Geometry: final body of the model. Coordinates: model frame, mm. Give positions to 0.01 mm unless a question says otherwise; leave off trailing zeros. Write each loop counter-clockwise with the first axis right and the second up, starting at its lowest first coordinate (ties: lowest second). Pieces come first, ordered by that corner, then holes. Notation, with made-up numbers: (-19, 68) -> (33, 68) arc R27 cw to (33, 84) -> close; hole circle Ø3 at (-16.5, 31.25). An arc over 180 degrees is marked (long way). Answer as a JSON object with one key per item and string values.
from build123d import *

# Parameters (mm, degrees)
SKETCH_1_R      = 1.5
EXTRUDE_1_DEPTH = 3


with BuildPart() as part:
    # 草图1 → 凸台-拉伸1 (new body)
    with BuildSketch(Plane.XY):
        with BuildLine():
            Line((116, -441), (116, -336.18))
            ThreePointArc((116, -336.18), (118, -332.18), (116, -328.18))
            Line((116, -328.18), (116, -4))
            ThreePointArc((116, -4), (116.535533906, 3.535533906), (109, 3))
            Line((109, 3), (106, 3))
            Line((106, 3), (106, -21.645755349))
            Line((106, -21.645755349), (7, -21.645755349))
            Line((7, -21.645755349), (7, 3))
            Line((7, 3), (4, 3))
            ThreePointArc((4, 3), (-3.535533906, 3.535533906), (-3, -4))
            Line((-3, -4), (-3, -328.18))
            ThreePointArc((-3, -328.18), (-5, -332.18), (-3, -336.18))
            Line((-3, -336.18), (-3, -441))
            ThreePointArc((-3, -441), (-3.535533906, -448.535533906), (4, -448))
            Line((4, -448), (109, -448))
            ThreePointArc((109, -448), (116.535533906, -448.535533906), (116, -441))
        make_face()
        Circle(SKETCH_1_R, mode=Mode.SUBTRACT)
        with Locations((113, 0)):
            Circle(SKETCH_1_R, mode=Mode.SUBTRACT)
        with Locations((113, -445)):
            Circle(SKETCH_1_R, mode=Mode.SUBTRACT)
        with Locations((0, -445)):
            Circle(SKETCH_1_R, mode=Mode.SUBTRACT)
        with Locations((0, -332.18)):
            Circle(SKETCH_1_R, mode=Mode.SUBTRACT)
        with Locations((113, -332.18)):
            Circle(SKETCH_1_R, mode=Mode.SUBTRACT)
        with BuildLine():
            Line((101, -37), (101, -353.3033361))
            ThreePointArc((101, -353.3033361), (98.371573189, -356.280236059), (95.092044423, -354.040760242))
            Line((95.092044423, -354.040760242), (15.005818776, -38.229040236))
            ThreePointArc((15.005818776, -38.229040236), (15.906197954, -33.929592957), (19.852411404, -32))
            Line((19.852411404, -32), (96, -32))
            ThreePointArc((96, -32), (99.535533906, -33.464466094), (101, -37))
        make_face(mode=Mode.SUBTRACT)
        with BuildLine():
            Line((20.846592628, -97.875461369), (106.279422364, -434.770959764))
            ThreePointArc((106.279422364, -434.770959764), (105.379043186, -439.070407043), (101.432829737, -441))
            Line((101.432829737, -441), (16, -441))
            ThreePointArc((16, -441), (12.464466094, -439.535533906), (11, -436))
            Line((11, -436), (11, -99.104501604))
            ThreePointArc((11, -99.104501604), (15.380711351, -94.143001673), (20.846592628, -97.875461369))
        make_face(mode=Mode.SUBTRACT)
    extrude(amount=EXTRUDE_1_DEPTH)


solid = part.part
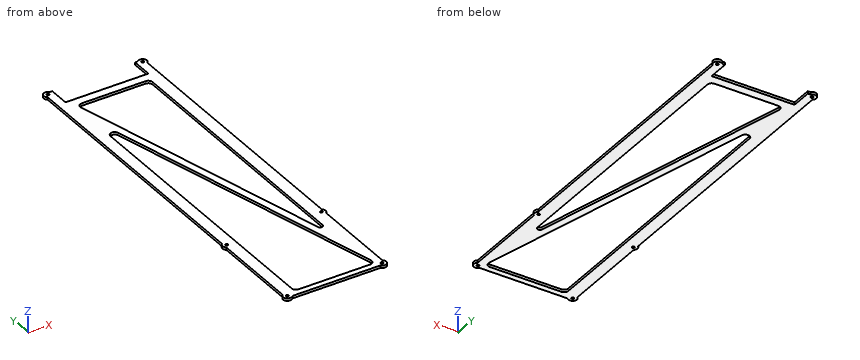
Q1. Cut plane D-D (y = -60). Return the cut outline in (x, z).
Values:
{"outline": "(-3, 0) -> (20.53, 0) -> (20.53, 3) -> (-3, 3) -> close; (101, 0) -> (116, 0) -> (116, 3) -> (101, 3) -> close"}
Q2. Cut plane B-B (y = -177.5). Return the cut outline in (x, z), and give its area (3 significant figures).
Values:
{"outline": "(-3, 0) -> (11, 0) -> (11, 3) -> (-3, 3) -> close; (41.04, 0) -> (50.32, 0) -> (50.32, 3) -> (41.04, 3) -> close; (101, 0) -> (116, 0) -> (116, 3) -> (101, 3) -> close", "area": "115 mm²"}
Q3. Material intervals for L1, parallel to Y at x = 0, z = 0.75; L2, parallel to X at y = -445, z = 0.95; L3, parallel to X at y = -113, z = 1, sorted ascending. Write a range as from..to.
Values:
{"L1": "-450..-446.5, -443.5..-333.68, -330.68..-1.5, 1.5..5", "L2": "-5..-1.5, 1.5..111.5, 114.5..118", "L3": "-3..11, 24.68..33.97, 101..116"}
Q4. First-contact query: P1, Ø1, axis at x = 12.5, z = 1, coming from the -Y side; P2, Ø1.8, axis at x = 113, y = 0, coming from the -Z side; P3, Ø0.9, axis at x = 107.5, z = 1, coming from the +Y side; P4, Ø1.5, axis at y = -239, z = 1, coming from the -X side. Flat tips, straight axial feed; report the tip coordinate or a pass-through.
Values:
{"P1": "y = -448", "P2": "through", "P3": "y = 3", "P4": "x = -3"}
Q5. Cut plane C-C (x = 32.5). Return the cut outline in (y, z), and give its area (3 significant figures).
Values:
{"outline": "(-448, 0) -> (-441, 0) -> (-441, 3) -> (-448, 3) -> close; (-143.83, 0) -> (-107.22, 0) -> (-107.22, 3) -> (-143.83, 3) -> close; (-32, 0) -> (-21.65, 0) -> (-21.65, 3) -> (-32, 3) -> close", "area": "162 mm²"}
Q6. Cut plane A-A (z = 1.6). State how many separate pieces and enclosed holes the cut face has, and give its area (3 significant figures).
Values:
{"separate pieces": "1", "enclosed holes": "8", "area": "17,900 mm²"}
